Job drawing, mm, ordinate dimensions from the low corner. One solid piece. A direction names the side the tool comes from. Give positions to 0.01 mm unless a question says otherwise; leave off trailing zeros. Write each loop counter-clockwise with the first axis right and the second up, starting at its lowest first coordinate (ties: lowest second). Pieces come first, ordered by that corner, then holes. Notation, with made-up numbers: M -3.5,68 L 16.5,68 A28 cw 16.5,96 Z; hole C 5,-22 d7. An arc over 180 degrees is marked long. Use a Markdown table: item, result.
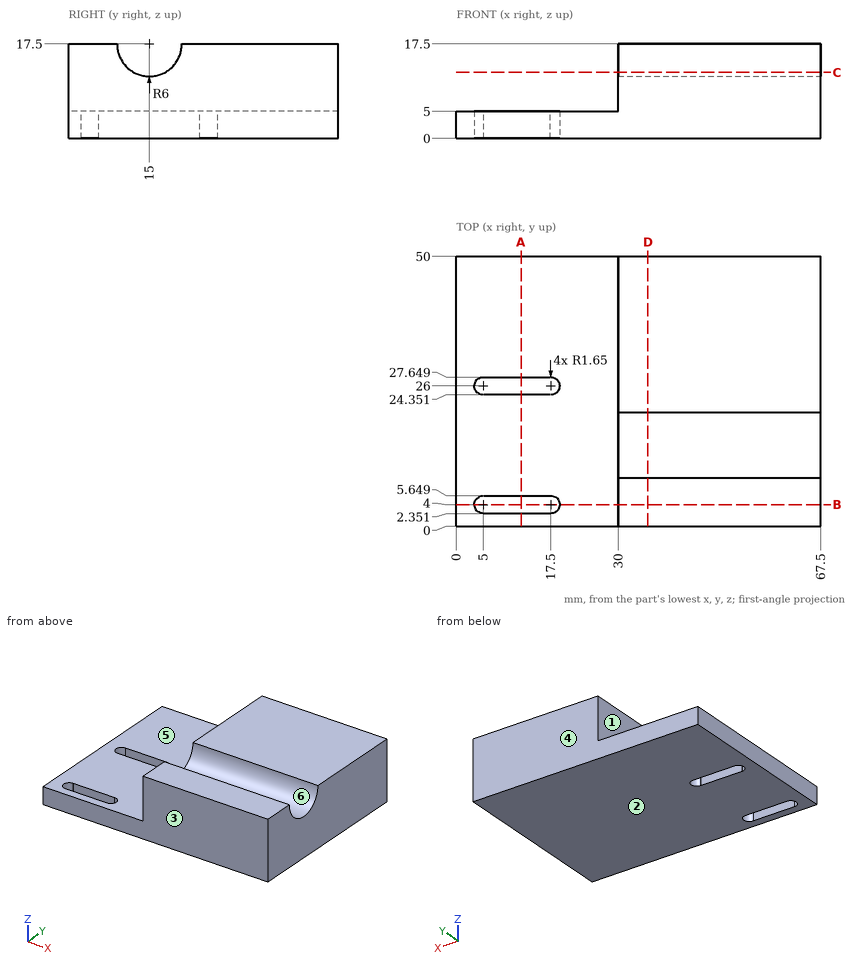
1. Cut at C-C, the plane z = 12.25. Give the cut face in (x, y), then the cut area to 3 significant figures.
Findings below:
| item | result |
|---|---|
| outline | M 30,0 L 67.5,0 L 67.5,12.1 L 30,12.1 Z; M 30,17.9 L 67.5,17.9 L 67.5,50 L 30,50 Z |
| area | 1,660 mm2 |
2. Cut at A-A, the plane x = 12. Give the cut face in (y, z).
Findings below:
| item | result |
|---|---|
| outline | M 0,0 L 2.35,0 L 2.35,5 L 0,5 Z; M 5.65,0 L 24.35,0 L 24.35,5 L 5.65,5 Z; M 27.65,0 L 50,0 L 50,5 L 27.65,5 Z |
3. Drill centre lines: L1, parallel to X at y = 38.5, z = 15; L2, parallel to Z at x = 8, y = 33; L3, parallel to Y at x = 60, z = 15. Where is each one in solid material? Low to high.
Findings below:
| item | result |
|---|---|
| L1 | 30 to 67.5 |
| L2 | 0 to 5 |
| L3 | 0 to 9.55, 20.45 to 50 |
4. Tool access for the marked faces 1 and 2: list every direction of +Z, -Z, +X, -X, +Y, -Y with a clear straight run to the whole face (end or side of a thin tool).
Findings below:
| item | result |
|---|---|
| face 1 | +Z, -X, +Y, -Y |
| face 2 | -Z, +X, -X, +Y, -Y |
5. Cut at D-D, the plane x = 35.5. Give the cut face in (y, z).
Findings below:
| item | result |
|---|---|
| outline | M 0,0 L 50,0 L 50,17.5 L 21,17.5 A6 cw 9,17.5 L 0,17.5 Z |
6. Drop flat-ended pins along their axis: P1, Ø9, axis at x = 20, y = 19.5, coming from the +Z side; P2, Ø4, axis at y = 34.5, z = 9.5, coming from the -X side. Give the stop position or say it passes through.
Findings below:
| item | result |
|---|---|
| P1 | z = 5 |
| P2 | x = 30 |
7. Cut at B-B, the plane y = 4. Give the cut face in (x, z).
Findings below:
| item | result |
|---|---|
| outline | M 0,0 L 3.35,0 L 3.35,5 L 0,5 Z; M 19.15,0 L 67.5,0 L 67.5,17.5 L 30,17.5 L 30,5 L 19.15,5 Z |
8. Two-plate mould, pull along Y, no slides. Class the marked faces 3, 4, 5 and 6: released by +Y, released by -Y, zero draft, split by the parting line, or undercut.
Findings below:
| item | result |
|---|---|
| face 3 | released by -Y |
| face 4 | released by +Y |
| face 5 | zero draft |
| face 6 | undercut |
